```python
from build123d import *

# Parameters (mm, degrees)
SKETCH1_W           = 23.65
SKETCH1_H           = 40
BOSS_EXTRUDE1_DEPTH = 56.55
SKETCH2_W           = 16
SKETCH2_H           = 28.38
CUT_EXTRUDE1_DEPTH  = 62.137002911
SKETCH3_R           = 7
CUT_EXTRUDE2_DEPTH  = 6.2205
SKETCH6_R           = 3.025
CUT_EXTRUDE4_DEPTH  = 8
SKETCH4_W           = 11.968
SKETCH4_H           = 10
BOSS_EXTRUDE2_DEPTH = 28.38
SKETCH5_W           = 12.292
SKETCH5_H           = 28.38
CUT_EXTRUDE3_DEPTH  = 6.2205
FILLET5_R           = 2
SKETCH9_W           = 8
SKETCH9_H           = 11
BOSS_EXTRUDE3_DEPTH = 16
SKETCH8_R           = 2.7
CUT_EXTRUDE6_DEPTH  = 6
SKETCH7_R           = 2.7
CUT_EXTRUDE5_DEPTH  = 8
FILLET4_R           = 2


with BuildPart() as part:
    # Sketch1 → Boss-Extrude1 (new body)
    with BuildSketch(Plane.XY):
        Rectangle(SKETCH1_W, SKETCH1_H)
    extrude(amount=BOSS_EXTRUDE1_DEPTH)

    # Sketch2 → Cut-Extrude1 (cut, through all)
    with BuildSketch(Plane.XY.offset(56.55)):
        with Locations((-2.3955, -5.81)):
            Rectangle(SKETCH2_W, SKETCH2_H)
    extrude(amount=-CUT_EXTRUDE1_DEPTH, mode=Mode.SUBTRACT)

    # Sketch3 → Cut-Extrude2 (cut)
    with BuildSketch(Plane(origin=(11.825, 0, 0), x_dir=(0, 0, -1), z_dir=(1, 0, 0))):
        with Locations(Location((-28.275, 0, 0), (0, 0, 90))):
            Circle(SKETCH3_R)
    extrude(amount=-CUT_EXTRUDE2_DEPTH, mode=Mode.SUBTRACT)

    # Sketch6 → Cut-Extrude4 (cut)
    with BuildSketch(Plane(origin=(11.825, 0, 0), x_dir=(0, 0, -1), z_dir=(1, 0, 0))):
        with Locations(Location((-28.275, 12, 0), (0, 0, 90))):
            Circle(SKETCH6_R)
        with Locations(Location((-28.275, -12, 0), (0, 0, 90))):
            Circle(SKETCH6_R)
    extrude(amount=-CUT_EXTRUDE4_DEPTH, mode=Mode.SUBTRACT)

    # Sketch4 → Boss-Extrude2 (add)
    with BuildSketch(Plane.XZ.offset(-8.38)):
        with Locations((-0.3795, 51.55)):
            Rectangle(SKETCH4_W, SKETCH4_H)
    extrude(amount=BOSS_EXTRUDE2_DEPTH)

    # Sketch5 → Cut-Extrude3 (cut)
    with BuildSketch(Plane(origin=(11.825, 0, 0), x_dir=(0, 0, -1), z_dir=(1, 0, 0))):
        with Locations((-40.404, -5.81)):
            Rectangle(SKETCH5_W, SKETCH5_H)
    extrude(amount=-CUT_EXTRUDE3_DEPTH, mode=Mode.SUBTRACT)

    # Fillet5
    fillet5_edges = [part.edges().sort_by_distance(p)[0] for p in [
        (5.6045, 8.38, 17.129),
    ]]
    fillet(fillet5_edges, radius=FILLET5_R)

    # Sketch9 → Boss-Extrude3 (add)
    with BuildSketch(Plane(origin=(-10.3955, 0, 0), x_dir=(0, 0, -1), z_dir=(1, 0, 0))):
        with Locations((-4, -14.5)):
            Rectangle(SKETCH9_W, SKETCH9_H)
    extrude(amount=BOSS_EXTRUDE3_DEPTH)

    # Sketch8 → Cut-Extrude6 (cut)
    with BuildSketch(Plane(origin=(0, 0, 0), x_dir=(-1, 0, 0), z_dir=(0, 0, -1))):
        with Locations((0, 14.19)):
            Circle(SKETCH8_R)
        with Locations((0, -14.5)):
            Circle(SKETCH8_R)
    extrude(amount=-CUT_EXTRUDE6_DEPTH, mode=Mode.SUBTRACT)

    # Sketch7 → Cut-Extrude5 (cut)
    with BuildSketch(Plane.XY.offset(56.55)):
        with Locations((2.73075, 12.5)):
            Circle(SKETCH7_R)
        with Locations((2.73075, -12.5)):
            Circle(SKETCH7_R)
    extrude(amount=-CUT_EXTRUDE5_DEPTH, mode=Mode.SUBTRACT)

    # Fillet4
    fillet4_edges = [part.edges().sort_by_distance(p)[0] for p in [
        (5.6045, -14.5, 8),
        (5.6045, -9, 4),
        (2.73075, -20, 46.55),
        (2.73075, 8.38, 46.55),
        (8.71475, 3.633691099, 34.258),
        (8.71475, -3.633691099, 34.258),
        (11.825, -20, 17.129),
        (11.825, 8.38, 40.404),
        (11.825, -11.816845549, 34.258),
        (11.825, 6.006845549, 34.258),
        (11.825, -5.81, 46.55),
        (8.71475, -20, 34.258),
        (11.825, -20, 51.55),
        (11.825, 20, 28.275),
    ]]
    fillet(fillet4_edges, radius=FILLET4_R)


solid = part.part
```
Work out the finished part from the listing and answer in its coordinate system (mm). A direction names the side the tool comes from. Give positions to 0.01 mm unless a question says otherwise; leave off trailing zeros. Loops run counter-clockwise (first coordinate to the right, second up) from the corner with the lowest first, then second, coordinate; pieces in that order, holes last. Notation, with made-up numbers: M -30,48.5 L 0,48.5 A17 cw 0,75.5 Z; hole C 23.25,-30 d10. An arc over 180 degrees is marked long. One line per item, written item: value. Start each with the question number.
1. This flat-tipped pin is pushed along its axis until it touches: P1, Ø4, axis at x = -6, z = 22.5, coming from the -Y side. Where does it stop, or does it pass through?
2. Find section B-B (z = 41). Give the vertices of the cut face in (x, y) (1 decimal).
3. Find section D-D (x = -3.75). Give the vertices of the cut face in (y, z).
4. Find the intervals of material crossed by probe 1 along Y at (x, z) = (0, 2.2); probe 2 along Z at (x, y) = (9.25, -12); probe 3 along Y at (x, z) = (-2.5, 7), in increasing order.
5. Find section A-A (x = -9.5). Give the vertices of the cut face in (y, z).
6. Determine the mould class of faces 6 (the face through (11.3, -5.6, 47.2)), 7 (the face through (0, -14, 6)), 8 (the face through (1.84, 7.81, 45.95)) for opening direction X: released by +X, released by -X, zero draft, split by the parting line, or undercut.
7. Which of the six approach directions +Z, -Z, +X, -X, +Y, -Y give full straight-line access (tool end or side, diameter ignored) to faces 1 (the face through (3, -12, 48.55)), 2 (the face through (-3, -15, 8)), 3 (the face through (1.62, -19.4, 47.12)), 4 (the face through (5, -8.43, 3.82)), 5 (the face through (5.604, -7, 17))?
8. Find section C-C (y = -3). State how many separate pieces and enclosed holes the cut face has, and give its area (3 significant figures).
Reported:
1. P1: stops at y = 8.38
2. outline: M -11.8,-20 L -10.4,-20 L -10.4,8.4 L 9.8,8.4 A2 ccw 11.8,10.4 L 11.8,18 A2 ccw 9.8,20 L -11.8,20 Z
3. outline: M -20,0 L -9,0 L -9,8 L -20,8 Z; M -20,48.55 A2 ccw -18,46.55 L 6.38,46.55 A2 cw 8.38,44.55 L 8.38,0 L 20,0 L 20,56.55 L -20,56.55 Z
4. probe 1: y = -20 to -17.2, -11.8 to -9, 8.38 to 11.49, 16.89 to 20
4. probe 2: z = 0 to 25.25, 31.3 to 34.26, 46.55 to 56.55
4. probe 3: y = -20 to -9, 8.38 to 20
5. outline: M -20,0 L -9,0 L -9,8 L -20,8 Z; M 8.38,0 L 20,0 L 20,56.55 L 8.38,56.55 Z
6. face 6: released by +X
6. face 7: undercut
6. face 8: zero draft
7. face 1: +Z
7. face 2: -Y
7. face 3: +X, -Y
7. face 4: -Z
7. face 5: none
8. separate pieces: 3
8. enclosed holes: 0
8. area: 398 mm²
